Verification items for this drawing (mm, ordinates from the low corner). A direction names the side the tool comes from. Round coordinates to 2 decimals unless told otherwise and drop trailing zeros. Order: outer loops, then holes, each group sorted by start corner. A loop starts at its lowest first (then second) coordinate and runs counter-clockwise, first axis right, second up. Notation, with made-up numbers: (52, -26.5) -> (103, -26.5) arc R26 ccw to (103, 1.5) -> close; hole circle Ø7 at (-35.5, -28.5). An arc over 180 degrees is marked (long way). Answer in a Markdown table with one row per item.
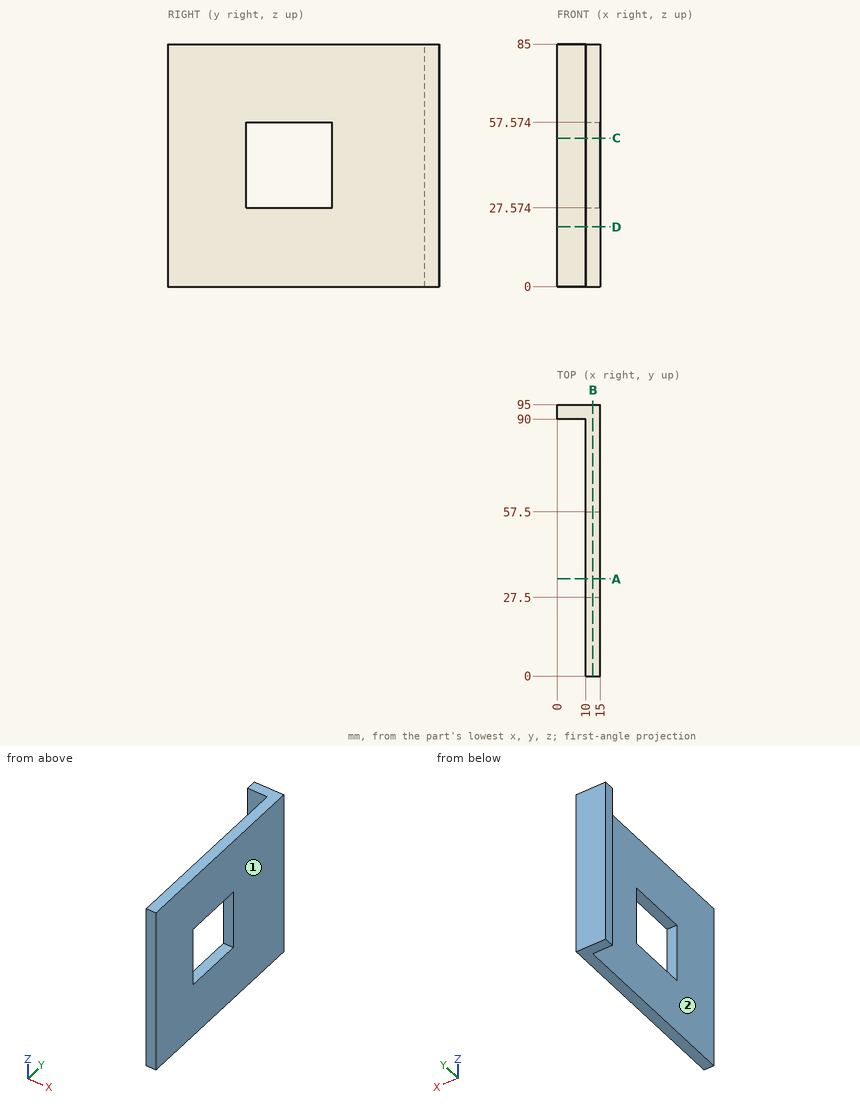
Item 1: Cross-section at B-B (x = 12.5). Record the boundary of the cut face in (y, z), and give its area (4 significant figures).
Result sheet:
| item | result |
|---|---|
| outline | (0, 0) -> (95, 0) -> (95, 85) -> (0, 85) -> close; hole (27.5, 27.57) -> (57.5, 27.57) -> (57.5, 57.57) -> (27.5, 57.57) -> close |
| area | 7,175 mm^2 |
Item 2: Cross-section at D-D (z = 21). Record the boundary of the cut face in (x, y), and give its area (3 significant figures).
Result sheet:
| item | result |
|---|---|
| outline | (0, 90) -> (10, 90) -> (10, 0) -> (15, 0) -> (15, 95) -> (0, 95) -> close |
| area | 525 mm^2 |
Item 3: Cross-section at A-A (y = 34). Record the boundary of the cut face in (x, z).
Result sheet:
| item | result |
|---|---|
| outline | (10, 0) -> (15, 0) -> (15, 27.57) -> (10, 27.57) -> close; (10, 57.57) -> (15, 57.57) -> (15, 85) -> (10, 85) -> close |
Item 4: Depth check by flat-ended pin: P1, Ø12, axis at y = 14, z = 28.5, coming from the -X side; P2, Ø5, axis at x = 6.5, z = 44.5, coming from the -Y side. Enter the tip coordinate at first touch or a pass-through.
Result sheet:
| item | result |
|---|---|
| P1 | stops at x = 10 |
| P2 | stops at y = 90 |
Item 5: Cross-section at C-C (z = 52). Record the boundary of the cut face in (x, y).
Result sheet:
| item | result |
|---|---|
| outline | (0, 90) -> (10, 90) -> (10, 57.5) -> (15, 57.5) -> (15, 95) -> (0, 95) -> close; (10, 0) -> (15, 0) -> (15, 27.5) -> (10, 27.5) -> close |
Item 6: Scan lines: line 1 (Y direction, x = 13.5, z = 44.5); line 2 (Z direction, x = 13, y = 40); line 3 (X direction, y = 46, z = 74). Record each from-to range of solid material in increasing order. Write a range as [from, to].
Result sheet:
| item | result |
|---|---|
| line 1 | y = [0, 27.5], [57.5, 95] |
| line 2 | z = [0, 27.57], [57.57, 85] |
| line 3 | x = [10, 15] |
Item 7: Set-up check for the marked faces 1 and 2: record each of +Z, -Z, +X, -X, +Y, -Y from which the full face is reachable in a straight line by a thin tool's end or side.
Result sheet:
| item | result |
|---|---|
| face 1 | +Z, -Z, +X, +Y, -Y |
| face 2 | +Z, -Z, -X, -Y |
